```python
from build123d import *

# Parameters (mm, degrees)
SKETCH1_R                      = 4.125
BOSS_EXTRUDE1_DEPTH            = 20
FILLET2_R                      = 5
FILLET3_R                      = 5
FILLET4_R                      = 6
FILLET5_R                      = 6
FILLET6_R                      = 2
FILLET7_R                      = 3
FILLET10_R                     = 2
F_8_0_199_DIAMETER_HOLE2_D     = 4
F_8_0_199_DIAMETER_HOLE3_D     = 4
SKETCH12_W                     = 2
SKETCH12_H                     = 41.945563192
SKETCH16_W                     = 2
SKETCH16_H                     = 41.945563192
F_8_0_199_DIAMETER_HOLE8_D     = 3.000000096
F_8_0_199_DIAMETER_HOLE8_DEPTH = 4
F_8_0_199_DIAMETER_HOLE8_TIP   = 0.901290957


with BuildPart() as part:
    # Sketch1 → Boss-Extrude1 (new body)
    with BuildSketch(Plane(origin=(0, 0, 0), x_dir=(1, 0, 0), z_dir=(0, 1, 0))):
        with BuildLine():
            Line((-28.643593539, -10.537386441), (-38.169872981, -27.037386441))
            Line((-38.169872981, -27.037386441), (-42.5, -24.537386441))
            Line((-42.5, -24.537386441), (-14.5, 23.960036171))
            Line((-14.5, 23.960036171), (-31.820508076, 33.960036171))
            ThreePointArc((-31.820508076, 33.960036171), (0, 50.621689136), (31.820508076, 33.960036171))
            Line((31.820508076, 33.960036171), (14.5, 23.960036171))
            Line((14.5, 23.960036171), (42.5, -24.537386441))
            Line((42.5, -24.537386441), (38.169872981, -27.037386441))
            Line((38.169872981, -27.037386441), (28.643593539, -10.537386441))
            Line((28.643593539, -10.537386441), (-28.643593539, -10.537386441))
        make_face()
        with Locations((19.660254038, 35.022213998)):
            Circle(SKETCH1_R, mode=Mode.SUBTRACT)
        with Locations((-19.660254038, 35.022213998)):
            Circle(SKETCH1_R, mode=Mode.SUBTRACT)
        Polygon((-12.0447733, 18.212613559), (-26.47853003, -6.787386441), (-7.5, -6.787386441), (-3.75, -2.037386441), (3.75, -2.037386441), (7.5, -6.787386441), (26.47853003, -6.787386441), (12.0447733, 18.212613559), (3.75, 10.462613559), (-3.75, 10.462613559), align=None, mode=Mode.SUBTRACT)
        Polygon((-9.999491924, 47.962613559), (10.000508076, 47.962613559), (10.000508076, 39.587613559), (6.750508076, 39.587613559), (6.750508076, 36.337613559), (10.000508076, 36.337613559), (10.000508076, 27.962613559), (-9.999491924, 27.962613559), (-9.999491924, 36.337613559), (-6.749491924, 36.337613559), (-6.749491924, 39.587613559), (-9.999491924, 39.587613559), align=None, mode=Mode.SUBTRACT)
    extrude(amount=BOSS_EXTRUDE1_DEPTH)

    # Fillet2
    fillet2_edges = [part.edges().sort_by_distance(p)[0] for p in [
        (-28.643593539, 10, 10.537386441),
    ]]
    fillet(fillet2_edges, radius=FILLET2_R)

    # Fillet3
    fillet3_edges = [part.edges().sort_by_distance(p)[0] for p in [
        (28.643593539, 10, 10.537386441),
    ]]
    fillet(fillet3_edges, radius=FILLET3_R)

    # Fillet4
    fillet4_edges = [part.edges().sort_by_distance(p)[0] for p in [
        (-26.47853003, 10, 6.787386441),
    ]]
    fillet(fillet4_edges, radius=FILLET4_R)

    # Fillet5
    fillet5_edges = [part.edges().sort_by_distance(p)[0] for p in [
        (26.47853003, 10, 6.787386441),
    ]]
    fillet(fillet5_edges, radius=FILLET5_R)

    # Fillet6
    fillet6_edges = [part.edges().sort_by_distance(p)[0] for p in [
        (-12.0447733, 10, -18.212613559),
        (12.0447733, 10, -18.212613559),
    ]]
    fillet(fillet6_edges, radius=FILLET6_R)

    # Fillet7
    fillet7_edges = [part.edges().sort_by_distance(p)[0] for p in [
        (-3.75, 10, -10.462613559),
        (-3.75, 10, 2.037386441),
        (3.75, 10, 2.037386441),
        (3.75, 10, -10.462613559),
    ]]
    fillet(fillet7_edges, radius=FILLET7_R)

    # Fillet10
    fillet10_edges = [part.edges().sort_by_distance(p)[0] for p in [
        (-38.169872981, 10, 27.037386441),
        (-42.5, 10, 24.537386441),
        (42.5, 10, 24.537386441),
        (38.169872981, 10, 27.037386441),
    ]]
    fillet(fillet10_edges, radius=FILLET10_R)

    # #8 (0.199) Diameter Hole2 (through all)
    with Locations(Plane(origin=(16.919872981, 0, -9.76869322), x_dir=(0.5, 0, 0.866025404), z_dir=(-0.866025404, 0, 0.5))):
        with Locations((33.417096231, 10)):
            Hole(F_8_0_199_DIAMETER_HOLE2_D / 2)

    # #8 (0.199) Diameter Hole3 (through all)
    with Locations(Plane(origin=(-16.919872981, 0, -9.76869322), x_dir=(0.5, 0, -0.866025404), z_dir=(0.866025404, 0, 0.5))):
        with Locations((-33.417096231, 10)):
            Hole(F_8_0_199_DIAMETER_HOLE3_D / 2)

    # Sketch12 → #8 (0.199) Diameter Hole5 (revolve, cut)
    with BuildSketch(Plane(origin=(17.292785365, 10, -9.122790024), x_dir=(0.5, 0, 0.866025404), z_dir=(0, 1, 0))):
        with Locations((1, 20.972781596)):
            Rectangle(SKETCH12_W, SKETCH12_H)
    revolve(axis=Axis((11.793524051, 10, -5.947790024), (0.866025404, 0, -0.5)), mode=Mode.SUBTRACT)

    # Sketch16 → #8 (0.199) Diameter Hole6 (revolve, cut)
    with BuildSketch(Plane(origin=(-17.292785365, 10, -9.122790024), x_dir=(0.5, 0, -0.866025404), z_dir=(0, 1, 0))):
        with Locations((1, 20.972781596)):
            Rectangle(SKETCH16_W, SKETCH16_H)
    revolve(axis=Axis((-11.793524051, 10, -5.947790024), (-0.866025404, 0, -0.5)), mode=Mode.SUBTRACT)

    # Sketch18 → #8 (0.199) Diameter Hole7 (revolve, cut)
    with BuildSketch(Plane(origin=(0.000508076, 10, -47.962613559), x_dir=(0, -1, 0), z_dir=(1, 0, 0))):
        Polygon((0, 0), (0, 31.2017212), (1.999999937, 30), (1.999999937, 0), align=None)
    revolve(axis=Axis((0.000508076, 10, -41.612613559), (0, 0, -1)), mode=Mode.SUBTRACT)

    # #8 (0.199) Diameter Hole8
    with Locations(Plane.XY.offset(10.537386441)):
        with Locations((-15.499957804, 14.75), (15.500042196, 14.75)):
            Hole(F_8_0_199_DIAMETER_HOLE8_D / 2, depth=F_8_0_199_DIAMETER_HOLE8_DEPTH)
            with Locations((0, 0, -(F_8_0_199_DIAMETER_HOLE8_DEPTH + F_8_0_199_DIAMETER_HOLE8_TIP / 2))):  # 118° drill point
                Cone(0, F_8_0_199_DIAMETER_HOLE8_D / 2, F_8_0_199_DIAMETER_HOLE8_TIP, mode=Mode.SUBTRACT)


solid = part.part
```
Design review of the part built by this model. Coordinates are the model's own, in mm. A direction names the side the tool comes from. Give positions to 0.01 mm unless a question says otherwise; leave off trailing zeros. Write each loop counter-clockwise with the first axis right and the second up, starting at its lowest first coordinate (ties: lowest second). Pieces come first, ordered by that corner, then holes. Notation, with made-up numbers: (-0.5, 79) - (24.5, 79) arc R19 cw to (24.5, 101) - close; hole circle Ø7 at (4.25, -25.75). An arc over 180 degrees is marked (long way). Return JSON: item names as keys, results as strings. Group by question number.
(1) We need section C-C, the plane z = -0.5. Give the boundary of the cut face in (x, y).
(2) We need section B-B, the plane y = 10. Give the number of separate pieces and of enclosed holes in the cut face, then the cut area to 3 significant figures.
(3) Mouldability with a two-part tool opening along Z and no side actions: class faces 1 (the flat face through (23.28, 9.86, -29.03)), 2 (the flat face through (0, 0, -12)), 3 (the flat face through (33.68, 7.64, 19.26)) as +Z half, -Z half, draft (parallel to the pull), parting line (faces both ways), or undercut.
(4) Insertion check: pin 1 (6.5 mm diameter, centred on y = 6.5, z = -45, fed in from -X); pin 2 (1.8 mm diameter, centred on x = 15.5, y = 14.75, fed in from +Z); pin 3 (12 mm diameter, centred on x = 2, z = -13.5, fed in from -Y); pin 4 (3.5 mm diameter, centred on x = -8, y = 14.5, fed in from -Z). Each pin has a flat end and moves straight along its axis. Give the tip position at first contact, or say it passes through.
(5) We need section A-A, the plane z = -43.5. Give the boundary of the cut face in (x, y).
(6) Machinability: for faces 4 (the cylindrical face through (28.23, 10.14, 11.19)), 5 (the flat face through (-12, 10, 6.787)), 6 (the cylindrical face through (18.75, 8.65, -11.67)), 7 (the flat face through (27.811, 9.86, -0.905)), which of the approach directions +Z, -Z, +X, -X, +Y, -Y give a long, thin tool a straight path to every point of the face, cutting with its end or side? Answer none if there is none.
(7) To check wall thickness, follow probe 1 along Z at (x, y) = (1, 2.5); probe 2 along Z at (x, y) = (-19.5, 19); probe 3 along Z at (x, y) = (-15.5, 3.75). State the ranges of each line that lie inside material, in increasing order.
Reported:
{
 "1": {"outline": "(-28.04, 0) - (-21.95, 0) - (-21.95, 20) - (-28.04, 20) - close; (21.95, 0) - (28.04, 0) - (28.04, 20) - (21.95, 20) - close"},
 "2": {"separate pieces": "4", "enclosed holes": "2", "area": "1,760 mm2"},
 "3": {"face 1": "undercut", "face 2": "draft", "face 3": "+Z half"},
 "4": {"pin 1": "stops at x = -24.66", "pin 2": "stops at z = -10.67", "pin 3": "stops at y = 0", "pin 4": "stops at z = -50.11"},
 "5": {"outline": "(-22.38, 0) - (-10, 0) - (-10, 20) - (-22.38, 20) - close; (10, 0) - (22.38, 0) - (22.38, 20) - (10, 20) - close"},
 "6": {"face 4": "+Z, +Y, -Y", "face 5": "+Y, -Y", "face 6": "none", "face 7": "+X, +Y, -Y"},
 "7": {"probe 1": "z = -50.61 to -47.96, -27.96 to -10.46, 2.04 to 10.54", "probe 2": "z = -45.35 to -39.14, -30.9 to -26.85, -15.3 to -5.3, 5.72 to 10.54", "probe 3": "z = -47.38 to -24.54, -22.23 to -12.23, 6.79 to 10.54"}
}
